Build history of the part. All positions in model axes, mm. A direction names the side the tool comes from. Round coordinates to 2 decimals unless told otherwise and drop trailing zeros. Write each loop counter-clockwise with the first axis right and the second up, starting at its lowest first coordinate (ties: lowest second). Pieces come first, ordered by that corner, then holes. Notation, with made-up numbers: (68, 41.5) - (92, 41.5) arc R28 ccw to (92, 64.5) - close; hole circle Ø3 at (29.25, 15). An arc over 180 degrees is marked (long way). One line per question, with ' | ' between items.
from build123d import *

# Parameters (mm, degrees)
F0_R     = 6
F1_DEPTH = 16
F2_R     = 3
F3_DEPTH = 4
F4_SIZE  = 0.25
F5_SIZE  = 1.5


with BuildPart() as f1:
    # F0 (on Front) → F1 (new body)
    with BuildSketch(Plane.XZ):
        Circle(F0_R)
    extrude(amount=-F1_DEPTH)

    # F2 (on face) → F3 (join)
    with BuildSketch(Plane.XZ):
        Circle(F2_R)
    extrude(amount=F3_DEPTH)

    # F4
    f4_edges = [f1.edges().sort_by_distance(p)[0] for p in [
        (-3, -4, 0),
    ]]
    chamfer(f4_edges, length=F4_SIZE)

    # F5
    f5_edges = [f1.edges().sort_by_distance(p)[0] for p in [
        (-6, 16, 0),
    ]]
    chamfer(f5_edges, length=F5_SIZE)


solid = f1.part
Q1. Which spindle directions (+Z, -Z, +X, -X, +Y, -Y) get a long thin tool onto all of the face, cutting with end or side? Do faces 1 (the flat face through (0, 16, 0)), 2 (the cylindrical face through (-3, -2, 0)). Say none if no direction does.
Found:
face 1: +Z, -Z, +X, -X, +Y | face 2: -Y
Q2. Saw through at B-B, the plane x = 0. List the corners of the cut face in (y, z), then the cut area to 3 significant figures.
Found:
outline: (-4, -2.75) - (-3.75, -3) - (0, -3) - (0, -6) - (14.5, -6) - (16, -4.5) - (16, 4.5) - (14.5, 6) - (0, 6) - (0, 3) - (-3.75, 3) - (-4, 2.75) - close | area: 214 mm^2
Q3. Saw through at A-A, the plane z = 0. List the corners of the cut face in (x, y).
Found:
outline: (-6, 0) - (-3, 0) - (-3, -3.75) - (-2.75, -4) - (2.75, -4) - (3, -3.75) - (3, 0) - (6, 0) - (6, 14.5) - (4.5, 16) - (-4.5, 16) - (-6, 14.5) - close
Q4. Drill centre lines: L1, parallel to Y at x = -0.25, z = 3.25; L2, parallel to Z at x = 0.25, y = 10.5; L3, parallel to Z at x = -5, y = 5.75. Where is each one in solid material? Low to high. Write a range as from..to.
Found:
L1: 0..16 | L2: -5.99..5.99 | L3: -3.32..3.32
Q5. Saw through at C-C, the plane y = 6.5. List the corners of the cut face in (x, z), then the cut area to 3 significant figures.
Found:
outline: circle Ø12 at (0, 0) | area: 113 mm^2
Q6. Drop flat-ended pins along their axis: pin 1 (4 mm diameter, centred on y = 6, z = 4.5, fed in from +X); pin 2 (3 mm diameter, centred on x = -3.5, y = 6, fed in from +Z). Give the stop position or say it passes through.
Found:
pin 1: x = 5.45 | pin 2: z = 5.66
